from build123d import *

# Parameters (mm, degrees)
F1_DEPTH = 12
F2_R     = 50.708657
F2_R_2   = 36.219288
F3_DEPTH = 25


with BuildPart() as f1:
    # F0 (on Top) → F1 (new body)
    with BuildSketch(Plane.XY):
        Polygon((34.48616, 22.330118), (-39.507132, 22.330118), (-39.507132, -43.471057), (37.921563, -42.414013), align=None)
    extrude(amount=F1_DEPTH)

    # F2 (on Top) → F3 (join)
    with BuildSketch(Plane.XY):
        with Locations((-3.831795, -12.02391)):
            Circle(F2_R)
        with Locations((-3.831795, -12.02391)):
            Circle(F2_R_2, mode=Mode.SUBTRACT)
    extrude(amount=F3_DEPTH)


solid = f1.part
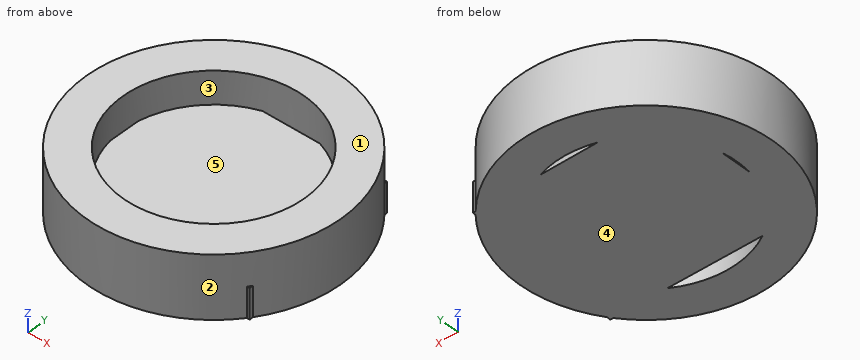
Here's how the part is built. I have some questions about the finished solid (model axes, mm). Face numbers are marked on the shaded views. A direction names the side the tool comes from. Coordinates: 2 decimals unless noted, no trailing zeros. Order: outer loops, then holes, each group sorted by start corner. A loop starts at its lowest first (then second) coordinate and runs counter-clockwise, first axis right, second up.
Item 1: If we section it at D-D on y = -19.5: List the corners of the cut face in (x, z) for me, plus the area to 3 significant figures.
Result sheet:
outline: (-53.99, 0) - (46.32, 0) - (46.32, 25) - (31.61, 25) - (31.61, 12) - (-39.27, 12) - (-39.27, 25) - (-53.99, 25) - close
area: 1,590 mm2
Item 2: For P1, Ø6, axis at y = 4, z = 12.5, coming from the +X side; P2, Ø1, axis at x = 16, z = 3, coming from the -Y side; P3, Ø1.5, axis at x = -16.5, z = 15, coming from the -Y side, each with a flat end and sliding along its axis, tell me the tip position at first contact or that it passes through.
Result sheet:
P1: stops at x = 45.18
P2: stops at y = -58.9
P3: stops at y = -61.31
Item 3: If we section it at C-C on x = 28.5: List the corners of the cut face in (y, z) for me.
Result sheet:
outline: (-51.09, 0) - (27.04, 0) - (27.04, 25) - (4.3, 25) - (4.3, 12) - (-28.35, 12) - (-28.35, 25) - (-51.09, 25) - close
Item 4: If we section it at B-B on x = -9.5: List the corners of the cut face in (y, z) for me, plus the area to 3 significant figures.
Result sheet:
outline: (-62.41, 0) - (-47.8, 0) - (-47.8, 25) - (-62.41, 25) - close; (-43.06, 0) - (22.33, 0) - (22.33, 12) - (-43.06, 12) - close; (23.75, 0) - (38.37, 0) - (38.37, 25) - (23.75, 25) - close
area: 1,520 mm2
Item 5: I need wall thicknesses on line 1 (Y direction, x = -5, z = 22.5); line 2 (Y direction, x = -7, z = 5); line 3 (X direction, y = -11, z = 4). Which ranges of each line are inside material? Lowest first, please.
Result sheet:
line 1: y = -62.72 to -48.22, 24.18 to 38.67
line 2: y = -62.63 to -48.1, -43.03 to 22.33, 24.06 to 38.59
line 3: x = -54.53 to -40.04, -39.51 to 46.87
Item 6: For the marked faces 4 and 5, which set-ups out of +Z, -Z, +X, -X, +Y, -Y let a thin tool reach every point of the face, with its end or its side?
Result sheet:
face 4: -Z, +X, -X, +Y, -Y
face 5: +Z
Item 7: If we mould it in two halves opening along Y, with no side actions, what happens to the marked faces 1, 2 and 3? For each: +Y half, -Y half, draft (parallel to the pull), parting line (faces both ways), or undercut.
Result sheet:
face 1: draft
face 2: parting line
face 3: undercut
Item 8: If we section it at A-A on z = 8.75: List the corners of the cut face in (x, y) for me, plus the area to 3 significant figures.
Result sheet:
outline: (33.47, 22.33) arc R50.71 ccw (long way) to (36.75, -42.43) - (37.92, -42.41) - (37.84, -40.91) arc R50.71 ccw to (34.55, 21.11) - (34.49, 22.33) - close; hole (-39.51, -18.28) - (-39.51, -5.77) arc R36.22 ccw to start; hole (-22.21, -43.23) arc R36.22 ccw to (15.39, -42.72) - close; hole (-15.31, 22.33) - (7.64, 22.33) arc R36.22 ccw to start
area: 7,910 mm2
